from build123d import *

# Parameters (mm, degrees)
SKETCH1_W            = 214
SKETCH1_H            = 214
BOSS_EXTRUDE1_DEPTH  = 1.51892
SKETCH2_W            = 204
SKETCH2_H            = 204
CUT_EXTRUDE1_DEPTH   = 1.51892
M3_CLEARANCE_HOLE1_D = 3.6


with BuildPart() as part:
    # Sketch1 → Boss-Extrude1 (new body)
    with BuildSketch(Plane(origin=(0, 0, 0), x_dir=(1, 0, 0), z_dir=(0, 1, 0))):
        Rectangle(SKETCH1_W, SKETCH1_H)
    extrude(amount=BOSS_EXTRUDE1_DEPTH)

    # Sketch2 → Cut-Extrude1 (cut)
    with BuildSketch(Plane(origin=(0, 1.51892, 0), x_dir=(1, 0, 0), z_dir=(0, 1, 0))):
        Rectangle(SKETCH2_W, SKETCH2_H)
    extrude(amount=-CUT_EXTRUDE1_DEPTH, mode=Mode.SUBTRACT)

    # M3 Clearance Hole1 (through all)
    with Locations(Plane(origin=(0, 1.51892, 0), x_dir=(1, 0, 0), z_dir=(0, 1, 0))):
        with Locations((-105, 105), (105, 105), (105, -105), (-105, -105)):
            Hole(M3_CLEARANCE_HOLE1_D / 2)


solid = part.part
Can you work these out from the model? Positions are in its coordinate system, mm. Give positions to 0.01 mm unless a question says otherwise; leave off trailing zeros. Write each loop counter-clockwise with the first axis right and the second up, starting at its lowest first coordinate (ties: lowest second). Pieces come first, ordered by that corner, then holes. Notation, with made-up numbers: M 12,13 L 28,13 A19 cw 28,38 Z; hole C -35.5,41 d9. An arc over 180 degrees is marked long. Answer in a Markdown table with one row per item. Add a question column.
Item 1: Please list where these lines run through material, in increasing order: L1, parallel to X at y = 1.15, z = 105; L2, parallel to X at y = 1.05, z = -4.
Item 2: Imagine slicing it at B-B, the plane z = -58. Write out the boundary of the cut face in (x, y), plus the area to 3 significant figures.
Item 3: Imagine slicing it at A-A, the plane x = 69. Write out the boundary of the cut face in (y, z).
Item 4: Imagine slicing it at C-C, the plane y = 1.2. Write out the boundary of the cut face in (x, z), plus the area to 3 significant figures.
Evaluation:
| question | item | result |
|---|---|---|
| 1 | L1 | x = -107 to -106.8, -103.2 to 103.2, 106.8 to 107 |
| 1 | L2 | x = -107 to -102, 102 to 107 |
| 2 | outline | M -107,0 L -102,0 L -102,1.52 L -107,1.52 Z; M 102,0 L 107,0 L 107,1.52 L 102,1.52 Z |
| 2 | area | 15.2 mm² |
| 3 | outline | M 0,-107 L 1.52,-107 L 1.52,-102 L 0,-102 Z; M 0,102 L 1.52,102 L 1.52,107 L 0,107 Z |
| 4 | outline | M -107,-107 L 107,-107 L 107,107 L -107,107 Z; hole C -105,-105 d3.6; hole C -105,105 d3.6; hole M -102,-102 L 102,-102 L 102,102 L -102,102 Z; hole C 105,-105 d3.6; hole C 105,105 d3.6 |
| 4 | area | 4,140 mm² |
